Study the drawing (mm; zero at the part's minimum x, y, z) and answer. A direction names the side the tool comes from. Coordinates: 2 decimals unless noted, no trailing zeros. Loops run counter-clockwise (first coordinate to the right, second up) from the corner with the lowest first, then second, coordinate; pieces in that order, holes last. Notation, with made-up numbers: M -23.75,-15.5 L -13.75,-15.5 A18 cw -13.75,-5.5 Z; hole C 29.25,46 d7. An arc over 180 degrees is marked long. Use one line per item in the form item = value. Start each with the question number.
1. The part is cut by section A-A (z = 21.4). Give the vertices of the cut face in (x, y), plus the area to 3 significant figures.
2. Flat-ended cylindrical pins translate along their axes: pin 1 (8 mm diameter, centred on x = 28.5, z = 22, fed in from +Y); pin 2 (7 mm diameter, centred on x = 21, y = 15.5, fed in from -Z); pin 3 (2.5 mm diameter, centred on y = 12.5, z = 32.5, fed in from +X). Find the tip coordinate at first contact, or state that the pin passes through.
3. The part is cut by section D-D (y = 23.75). Give the vertices of the cut face in (x, z), plus the area to 4 significant figures.
4. The part is cut by section C-C (z = 36). Give the vertices of the cut face in (x, y), plus the area to 3 significant figures.
5. The part is cut by section B-B (x = 12.5). Give the vertices of the cut face in (y, z), plus the area to 4 significant figures.
6. A tool of negligible diameter and unlimited length cuts with its end or side. For the marked faces 1 and 2, from which of +Z, -Z, +X, -X, +Y, -Y can it reach the whole face along a straight path? Write none if from no direction.
7. Find the intervals of material crossed by probe 1 along X at (y, z) = (12.25, 37); probe 2 along Y at (x, z) = (7.5, 6); probe 3 along X at (y, z) = (0.7, 21.4), in increasing order. Write a range as [from, to].
8. For a pull along X with two mould halves and no side action, classify the marked faces 3, 4 and 5 as released by +X, released by -X, zero draft, split by the parting line, or undercut.
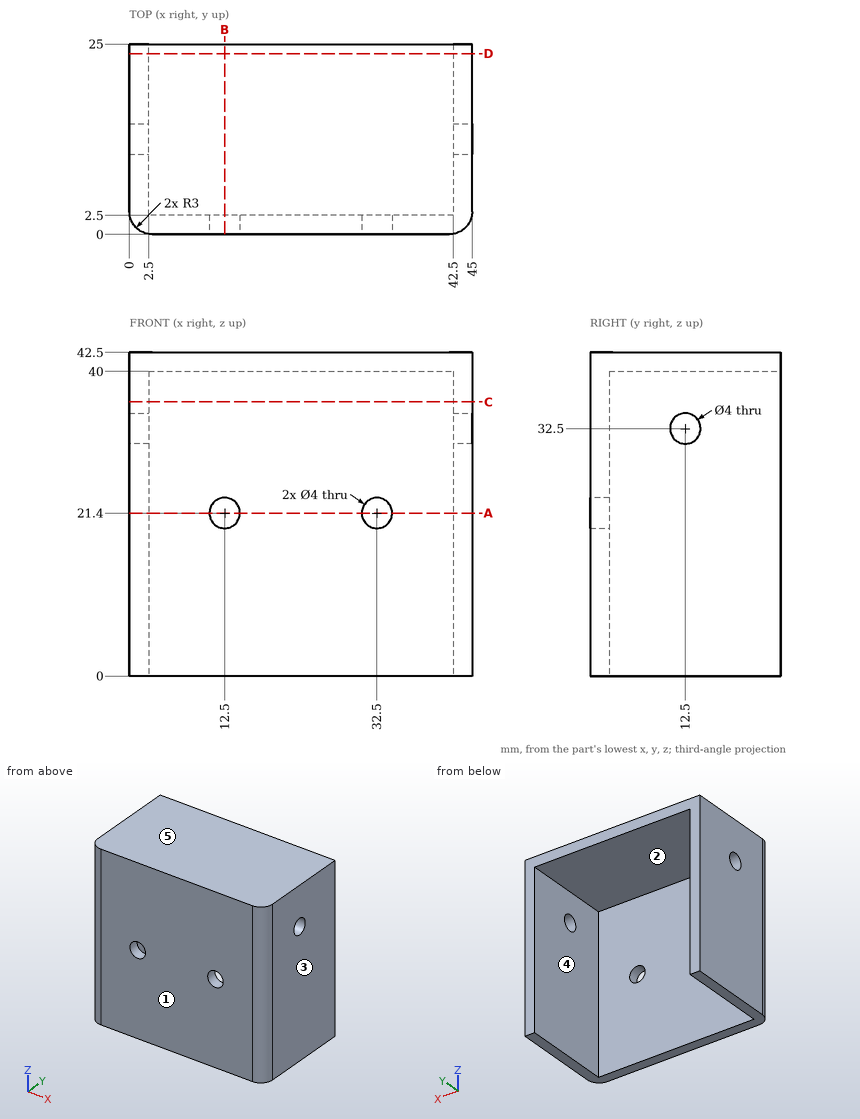
Computed values:
q1.outline = M 0,3 A3 ccw 3,0 L 10.5,0 L 10.5,2.5 L 2.5,2.5 L 2.5,25 L 0,25 Z; M 14.5,0 L 30.5,0 L 30.5,2.5 L 14.5,2.5 Z; M 34.5,0 L 42,0 A3 ccw 45,3 L 45,25 L 42.5,25 L 42.5,2.5 L 34.5,2.5 Z
q1.area = 201 mm²
q2.pin_1 = 2.5
q2.pin_2 = 40
q2.pin_3 = through
q3.outline = M 0,0 L 2.5,0 L 2.5,40 L 42.5,40 L 42.5,0 L 45,0 L 45,42.5 L 0,42.5 Z
q3.area = 312.5 mm²
q4.outline = M 0,3 A3 ccw 3,0 L 42,0 A3 ccw 45,3 L 45,25 L 42.5,25 L 42.5,2.5 L 2.5,2.5 L 2.5,25 L 0,25 Z
q4.area = 221 mm²
q5.outline = M 0,0 L 2.5,0 L 2.5,19.4 L 0,19.4 Z; M 0,23.4 L 2.5,23.4 L 2.5,40 L 25,40 L 25,42.5 L 0,42.5 Z
q5.area = 152.5 mm²
q6.face_1 = +Z, -Z, +X, -X, -Y
q6.face_2 = -Z, +Y
q7.probe_1 = [0, 2.5], [42.5, 45]
q7.probe_2 = [0, 2.5]
q7.probe_3 = [1.07, 10.5], [14.5, 30.5], [34.5, 43.93]
q8.face_3 = released by +X
q8.face_4 = undercut
q8.face_5 = zero draft
